Work out the finished part from the listing and answer in its coordinate system (mm). Face numbers are marked on the shaded views. A direction names the side the tool comes from. Coordinates: 2 decimals unless noted, no trailing zeros. Loops run counter-clockwise (first coordinate to the right, second up) from the corner with the lowest first, then second, coordinate; pieces in that order, holes last. Notation, with made-up numbers: (48, -22.5) -> (65, -22.5) arc R25 cw to (65, -4.5) -> close; hole circle Ø10 at (89, 87). An arc over 180 degrees is marked (long way). Use a Markdown table: item, result.
from build123d import *

# Parameters (mm, degrees)
BOSS_EXTRUDE1_DEPTH = 2
FILLET1_R           = 3
FILLET2_R           = 2
SKETCH3_R           = 1.5
CUT_EXTRUDE1_DEPTH  = 2
BOSS_EXTRUDE2_START = 1
BOSS_EXTRUDE2_DEPTH = 1
SKETCH3_5_R         = 1
BOSS_EXTRUDE3_DEPTH = 4


with BuildPart() as part:
    # Sketch1 → Boss-Extrude1 (new body)
    with BuildSketch(Plane.XY):
        Polygon((0, 0), (0, 15), (14, 15), (14, 11), (24, 11), (24, 13), (32, 13), (32, 11), (39, 11), (39, 0), align=None)
    extrude(amount=BOSS_EXTRUDE1_DEPTH)

    # Fillet1
    fillet1_edges = [part.edges().sort_by_distance(p)[0] for p in [
        (0, 0, 1),
        (0, 15, 1),
        (14, 15, 1),
        (39, 11, 1),
        (39, 0, 1),
    ]]
    fillet(fillet1_edges, radius=FILLET1_R)

    # Fillet2
    fillet2_edges = [part.edges().sort_by_distance(p)[0] for p in [
        (32, 11, 1),
        (24, 11, 1),
        (14, 11, 1),
    ]]
    fillet(fillet2_edges, radius=FILLET2_R - 0.0001)  # a hair under: the kernel refuses the full size

    # Sketch3 → Cut-Extrude1 (cut)
    with BuildSketch(Plane.XY.offset(2)):
        with Locations((7, 12)):
            Circle(SKETCH3_R)
        with Locations((11, 12)):
            Circle(SKETCH3_R)
        with Locations((36, 8)):
            Circle(SKETCH3_R)
    extrude(amount=-CUT_EXTRUDE1_DEPTH, mode=Mode.SUBTRACT)

    # Sketch3<4> → Boss-Extrude2 (add)
    with BuildSketch(Plane.XY.offset(2).offset(BOSS_EXTRUDE2_START)):
        with BuildLine():
            Line((0, 8), (0.25, 8))
            Line((0.25, 8), (0.25, 12))
            ThreePointArc((0.25, 12), (1.055456352, 13.944543648), (3, 14.75))
            Line((3, 14.75), (11, 14.75))
            ThreePointArc((11, 14.75), (12.739252713, 14.13014084), (13.694438717, 12.55))
            ThreePointArc((13.694438717, 12.55), (14.475954538, 11.257157494), (15.898979486, 10.75))
            Line((15.898979486, 10.75), (22, 10.75))
            ThreePointArc((22, 10.75), (23.590990258, 11.409009742), (24.25, 13))
            Line((24.25, 13), (24, 13))
            ThreePointArc((24, 13), (23.414213562, 11.585786438), (22, 11))
            Line((22, 11), (15.898979486, 11))
            ThreePointArc((15.898979486, 11), (14.634068421, 11.450806662), (13.939387691, 12.6))
            ThreePointArc((13.939387691, 12.6), (12.897366596, 14.323790008), (11, 15))
            Line((11, 15), (3, 15))
            ThreePointArc((3, 15), (0.878679656, 14.121320344), (0, 12))
            Line((0, 12), (0, 8))
        make_face()
        with BuildLine():
            ThreePointArc((3, 0.25), (1.055456352, 1.055456352), (0.25, 3))
            Line((0.25, 3), (0, 3))
            ThreePointArc((0, 3), (0.878679656, 0.878679656), (3, 0))
            Line((3, 0), (36, 0))
            ThreePointArc((36, 0), (38.121320344, 0.878679656), (39, 3))
            Line((39, 3), (39, 8))
            ThreePointArc((39, 8), (38.121320344, 10.121320344), (36, 11))
            Line((36, 11), (34, 11))
            ThreePointArc((34, 11), (32.585786438, 11.585786438), (32, 13))
            Line((32, 13), (31.75, 13))
            ThreePointArc((31.75, 13), (32.409009742, 11.409009742), (34, 10.75))
            Line((34, 10.75), (36, 10.75))
            ThreePointArc((36, 10.75), (37.944543648, 9.944543648), (38.75, 8))
            Line((38.75, 8), (38.75, 3))
            ThreePointArc((38.75, 3), (37.944543648, 1.055456352), (36, 0.25))
            Line((36, 0.25), (3, 0.25))
        make_face()
    extrude(amount=-BOSS_EXTRUDE2_DEPTH)

    # Sketch3<5> → Boss-Extrude3 (add)
    with BuildSketch(Plane.XY.offset(2)):
        with Locations(Location((3, 12, 0), (0, 0, 180))):
            Circle(SKETCH3_5_R)
        with Locations(Location((36, 3, 0), (0, 0, 180))):
            Circle(SKETCH3_5_R)
    extrude(amount=BOSS_EXTRUDE3_DEPTH)


solid = part.part
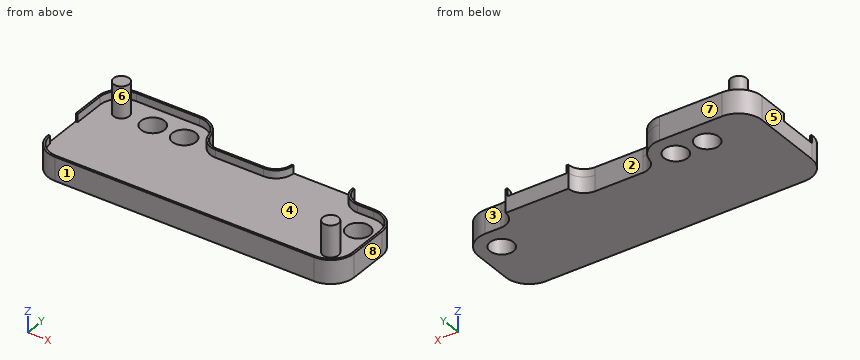
Q1. Section B-B on z = 5.5 is taken. Determine the outline of the cut face in (x, y).
Solved:
| item | result |
|---|---|
| outline | circle Ø2 at (3, 12); circle Ø2 at (36, 3) |
Q2. Section C-C on x = 19 is taken. Determine the outline of the cut face in (y, z).
Solved:
| item | result |
|---|---|
| outline | (0, 0) -> (11, 0) -> (11, 3) -> (10.75, 3) -> (10.75, 2) -> (0.25, 2) -> (0.25, 3) -> (0, 3) -> close |
Q3. Consider line 1 (Y direction, x = 11, z = 1.65); line 2 (X direction, y = 2.5, z = 2.5); line 3 (Z direction, x = 27.5, y = 7.5). Determine where each line is inside the solid, lowest interval first. Write a range as [from, to].
Solved:
| item | result |
|---|---|
| line 1 | [0, 10.5], [13.5, 15] |
| line 2 | [0.04, 0.3], [35.13, 36.87], [38.7, 38.96] |
| line 3 | [0, 2] |
Q4. For the marked faces 1, 2, 3, 4 and 5, determine the directions among +Z, -Z, +X, -X, +Y, -Y from which every point of the face is accessible in a straight line to the end or side of a thin tool.
Solved:
| item | result |
|---|---|
| face 1 | +Z, -Z, +X, -X, -Y |
| face 2 | +Z, -Z, +Y |
| face 3 | +Z, -Z, +X, +Y |
| face 4 | +Z |
| face 5 | +Z, -Z, -X, +Y, -Y |
Q5. Given pin 1 Ø3 at (x, y) = (19, 12) entering from +Z; pin 2 Ø1.6 at (x, z) = (35.5, 1.5) entering from +Y; pin 3 Ø1.5 at (y, z) = (12, 2) entering from +X, each flat-ended and moving along its own axis, determine where each tip first touches the part or whether it passes through.
Solved:
| item | result |
|---|---|
| pin 1 | z = 3 |
| pin 2 | y = 11 |
| pin 3 | x = 33.03 |
Q6. Section D-D on y = 4.5 is taken. Determine the outline of the cut face in (x, z).
Solved:
| item | result |
|---|---|
| outline | (0, 0) -> (39, 0) -> (39, 3) -> (38.75, 3) -> (38.75, 2) -> (0, 2) -> close |
Q7. Section A-A on x = 7 is taken. Determine the outline of the cut face in (y, z).
Solved:
| item | result |
|---|---|
| outline | (0, 0) -> (10.5, 0) -> (10.5, 2) -> (0.25, 2) -> (0.25, 3) -> (0, 3) -> close; (13.5, 0) -> (15, 0) -> (15, 3) -> (14.75, 3) -> (14.75, 2) -> (13.5, 2) -> close |
Q8. Determine the mould class of the marked faces 6, 7 and 8 for opening direction Y: pulls with the +Y half, pulls with the -Y half, needs draft (parallel to the pull), parting line crosses it, or undercut.
Solved:
| item | result |
|---|---|
| face 6 | undercut |
| face 7 | pulls with the +Y half |
| face 8 | needs draft |
